from build123d import *

# Parameters (mm, degrees)
BOSS_EXTRUDE1_DEPTH = 14
BOSS_EXTRUDE4_START = -60
SKETCH3_R           = 14
BOSS_EXTRUDE4_DEPTH = 104
SKETCH4_R           = 12.5
BOSS_EXTRUDE5_DEPTH = 60
SKETCH5_R           = 24
BOSS_EXTRUDE7_DEPTH = 18
SKETCH7_R           = 24
BOSS_EXTRUDE8_DEPTH = 18
CUT_EXTRUDE2_DEPTH  = 85
SKETCH10_R          = 12
CUT_EXTRUDE3_DEPTH  = 85


with BuildPart() as part:
    # Sketch2 → Boss-Extrude1 (new body, symmetric)
    with BuildSketch(Plane.XY):
        with BuildLine():
            Line((30, 14), (30, 32))
            Line((30, 32), (-30, 32))
            ThreePointArc((-30, 32), (-62, 0), (-30, -32))
            Line((-30, -32), (30, -32))
            Line((30, -32), (30, -14))
            Line((30, -14), (-30, -14))
            ThreePointArc((-30, -14), (-44, 0), (-30, 14))
            Line((-30, 14), (30, 14))
        make_face()
    extrude(amount=BOSS_EXTRUDE1_DEPTH, both=True)

    # Sketch3 → Boss-Extrude4 (add)
    with BuildSketch(Plane(origin=(0, 0, 0), x_dir=(0, 0, -1), z_dir=(1, 0, 0)).offset(BOSS_EXTRUDE4_START)):
        Circle(SKETCH3_R)
    extrude(amount=-BOSS_EXTRUDE4_DEPTH)

    # Sketch4 → Boss-Extrude5 (add)
    with BuildSketch(Plane.ZY.offset(164)):
        Circle(SKETCH4_R)
    extrude(amount=BOSS_EXTRUDE5_DEPTH)

    # Sketch5 → Boss-Extrude7 (add)
    with BuildSketch(Plane(origin=(0, 32, 0), x_dir=(1, 0, 0), z_dir=(0, 1, 0))):
        Circle(SKETCH5_R)
    extrude(amount=-BOSS_EXTRUDE7_DEPTH)

    # Sketch7 → Boss-Extrude8 (add)
    with BuildSketch(Plane.XZ.offset(32)):
        Circle(SKETCH7_R)
    extrude(amount=-BOSS_EXTRUDE8_DEPTH)

    # Sketch8 → Cut-Extrude2 (cut)
    with BuildSketch(Plane.XZ.offset(32)):
        with BuildLine():
            Line((19.49358869, -14), (30, -14))
            Line((30, -14), (30, 14))
            Line((30, 14), (19.49358869, 14))
            ThreePointArc((19.49358869, 14), (24, 0), (19.49358869, -14))
        make_face()
    extrude(amount=-CUT_EXTRUDE2_DEPTH, mode=Mode.SUBTRACT)

    # Sketch10 → Cut-Extrude3 (cut)
    with BuildSketch(Plane.XZ.offset(32)):
        Circle(SKETCH10_R)
    extrude(amount=-CUT_EXTRUDE3_DEPTH, mode=Mode.SUBTRACT)


solid = part.part
Input: part model. Units: mm. Frame: model coordinates. A direction names the side the tool comes from. Coordinates: 2 decimals unless noted, no trailing zeros. Loops run counter-clockwise (first coordinate to the right, second up) from the corner with the lowest first, then second, coordinate; pieces in that order, holes last. Notation, with made-up numbers: (50, -32) - (105, -32) arc R29 cw to (105, -12) - close; hole circle Ø2 at (36.5, 62). An arc over 180 degrees is marked (long way). Answer in a Markdown table with one row per item. Add a question column.
Item 1: Section query B-B on x = 0. Return the cut outline in (y, z), then the cut area to 3 significant figures.
Item 2: Section query D-D on y = 7. Return the cut outline in (x, z), then the cut area to 3 significant figures.
Item 3: Access query for faces 1 (the flat face through (-46, 0, 14)), 2 (the cylindrical face through (-111.272, -5.362, -12.932)), 3 (the flat face through (-224, 0, 0)), 4 (the flat face through (-15, 14, 0)), 5 (the flat face through (-15, 32, 0)). Directions: +Z, -Z, +X, -X, +Y, -Y. A direction counts if a zero-diameter tool reaches every point of the face in a straight line with its end or side. Return the directions, or none.
Item 4: Line query: line 1 along Z through (x, y) = (0, 24); line 2 along Y through (x, z) = (-13.5, 3); line 3 along X through (y, z) = (0, -1.5). Output: solid intervals per line, ascending. Write a range as [from, to].
Item 5: Contact query for flat-ended pins moving along their axis: P1, Ø0.9, axis at y = -12.5, z = -2, coming from the +X side; P2, Ø12, axis at x = -15, y = 12, coming from the +Z side; P3, Ø14.5, axis at x = 8, z = -6.5, coming from the +Y side; P4, Ø10, axis at x = -141, y = -20.5, coming from the +Z side. Output: stop coordinate, or through.
Item 6: Mould query, pull axis Z, two halves, no side actions, for faces 6 (the flat face through (-46, 0, -14)), 7 (the cylindrical face through (-11.99, 22.87, 0.53)), 8 (the flat face through (-164, 11.5, 5.3)). Classes: released by +Z, released by -Z, zero draft, split by the parting line, or undercut.
Item 7: Section query C-C on z = -17.5. Return the cut outline in (x, y), then the cut area to 3 significant figures.
Item 8: Section query A-A on z = 0. Return the cut outline in (x, y), then the cut area to 3 significant figures.
Recorded:
| question | item | result |
|---|---|---|
| 1 | outline | (-32, -24) - (-14, -24) - (-14, -12) - (-32, -12) - close; (-32, 12) - (-14, 12) - (-14, 24) - (-32, 24) - close; (14, -24) - (32, -24) - (32, -12) - (14, -12) - close; (14, 12) - (32, 12) - (32, 24) - (14, 24) - close |
| 1 | area | 864 mm^2 |
| 2 | outline | (-224, -10.36) - (-164, -10.36) - (-164, -12.12) - (-61.22, -12.12) - (-61.22, -14) - (-42.12, -14) - (-42.12, 14) - (-61.22, 14) - (-61.22, 12.12) - (-164, 12.12) - (-164, 10.36) - (-224, 10.36) - close |
| 2 | area | 4,270 mm^2 |
| 3 | face 1 | +Z, -X, +Y, -Y |
| 3 | face 2 | -X |
| 3 | face 3 | +Z, -Z, -X, +Y, -Y |
| 3 | face 4 | +Z, -Z, +X |
| 3 | face 5 | +Z, -Z, +X, -X, +Y |
| 4 | line 1 | [-24, -12], [12, 24] |
| 4 | line 2 | [-32, -14], [14, 32] |
| 4 | line 3 | [-224, -44] |
| 5 | P1 | x = -35.32 |
| 5 | P2 | z = 22.11 |
| 5 | P3 | y = 32 |
| 5 | P4 | through |
| 6 | face 6 | released by -Z |
| 6 | face 7 | undercut |
| 6 | face 8 | zero draft |
| 7 | outline | (-16.42, -32) - (16.42, -32) - (16.42, -14) - (-16.42, -14) - close; (-16.42, 14) - (16.42, 14) - (16.42, 32) - (-16.42, 32) - close |
| 7 | area | 1,180 mm^2 |
| 8 | outline | (-224, -12.5) - (-164, -12.5) - (-164, -14) - (-60, -14) - (-60, -11.14) arc R32 ccw to (-30, -32) - (-12, -32) - (-12, -14) - (-30, -14) arc R14 cw to (-30, 14) - (-12, 14) - (-12, 32) - (-30, 32) arc R32 ccw to (-60, 11.14) - (-60, 14) - (-164, 14) - (-164, 12.5) - (-224, 12.5) - close; (12, -32) - (24, -32) - (24, -14) - (12, -14) - close; (12, 14) - (24, 14) - (24, 32) - (12, 32) - close |
| 8 | area | 6,760 mm^2 |
